Read the model definition and answer for the solid it produces. Units are mm, in the model's axes. Give positions to 0.01 mm unless a question says otherwise; leave off trailing zeros. Order: outer loops, then holes, each group sorted by start corner. A loop starts at its lowest first (then second) coordinate and runs counter-clockwise, first axis right, second up. Notation, with made-up numbers: M 47,32 L 66,32 A32 cw 66,70 Z; hole C -23,84.25 d7. An arc over 180 degrees is marked long. One line per item, written item: value.
from build123d import *

# Parameters (mm, degrees)
SKETCH_1_W      = 100
SKETCH_1_H      = 100
SKETCH_1_R      = 2.5
EXTRUDE_1_DEPTH = 5


with BuildPart() as part:
    # 草图1 → 凸台-拉伸1 (new body)
    with BuildSketch(Plane(origin=(0, 0, 0), x_dir=(1, 0, 0), z_dir=(0, 1, 0))):
        Rectangle(SKETCH_1_W, SKETCH_1_H)
        Circle(SKETCH_1_R, mode=Mode.SUBTRACT)
        with Locations((16, 16)):
            Circle(SKETCH_1_R, mode=Mode.SUBTRACT)
    extrude(amount=EXTRUDE_1_DEPTH)


solid = part.part
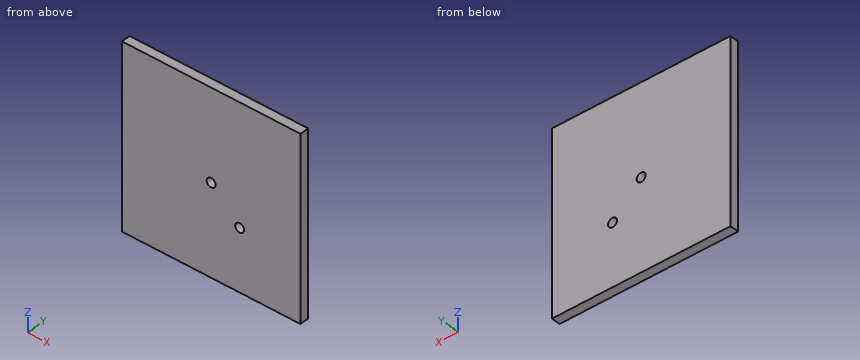
1) Consider probe 1 along X at (y, z) = (1.65, 0); probe 2 along X at (y, z) = (3.4, -16); probe 3 along Z at (x, y) = (16, 2.1). Determine where each line is inside the solid, lowest interval first.
Reported:
probe 1: x = -50 to -2.5, 2.5 to 50
probe 2: x = -50 to 13.5, 18.5 to 50
probe 3: z = -50 to -18.5, -13.5 to 50
2) This flat-tipped pin is pushed along its axis until it touches: pin 1 Ø4 at (x, z) = (0, 0) entering from +Y. Where does it stop, or does it pass through?
Reported:
pin 1: passes through
3) Find section B-B, the plane z = -16. Write down the section's boundary in (x, y).
Reported:
outline: M -50,0 L 13.5,0 L 13.5,5 L -50,5 Z; M 18.5,0 L 50,0 L 50,5 L 18.5,5 Z
4) Find section A-A, the plane x = 16. Write down the section's boundary in (y, z).
Reported:
outline: M 0,-50 L 5,-50 L 5,-18.5 L 0,-18.5 Z; M 0,-13.5 L 5,-13.5 L 5,50 L 0,50 Z
